Geometry: final body of the model. Coordinates: model frame, mm. Face numbers are marked on the shaded views. A direction names the side the tool comes from. Coordinates: 2 decimals unless noted, no trailing zeros. Order: outer loops, then holes, each group sorted by start corner. A loop starts at its lowest first (then second) coordinate and runs counter-clockwise, first axis right, second up. Notation, with made-up numbers: (64, -18) -> (95, -18) arc R30 ccw to (95, 8) -> close; hole circle Ø5 at (15, 56.5). An arc over 180 degrees is marked (long way). Answer in a Markdown table with one row per item. Add a question column.
1) Ray query, line 1 (Z direction, x = 45, y = 4); line 2 (X direction, y = 4.5, z = -26.5) (3 decimals); line 3 (Z direction, x = 63, y = 7.5). Return the intervals inside material, ascending. Write a range as from..to.
2) Section query A-A on x = 25. Return the cut outline in (y, z) (3 decimals).
3) Section query D-D on x = 48. Return the cut outline in (y, z) (3 decimals), then the cut area to 3 significant figures.
4) Section query B-B on y = 6.5. Return the cut outline in (x, z) (3 decimals), then the cut area to 3 significant figures.
5) Contact query for flat-ended pins moving along their axis: P1, Ø3.5, axis at y = 1, z = -11, coming from the -X side; P2, Ø2.5, axis at y = 1.5, z = -12, coming from the +X side; P3, Ø2.5, axis at x = 55.5, y = 1.5, coming from the +Z side; P4, Ø3.5, axis at y = 2.5, z = -13, coming from the -X side. Output: stop coordinate, or through.
6) Set-up query: the marked faces 1 and 2. Return all of +Z, -Z, +X, -X, +Y, -Y with unobstructed straight access to the full face (end or side cutting, diameter ignored); none if empty.
7) Section query C-C on z = -13. Return the cut outline in (x, y) (3 decimals), then the cut area to 3 significant figures.
8) Pull-direction query (Z, two-part tool) for the marked faces 3, 4 and 5; classes: +Z half, -Z half, draft (parallel to the pull), parting line (faces both ways), or undercut.
```python
from build123d import *

# Parameters (mm, degrees)
SKETCH1_W           = 72.39
SKETCH1_H           = 48.514
BOSS_EXTRUDE1_DEPTH = 8.636
SKETCH2_W           = 63.5
SKETCH2_H           = 40.64
CUT_EXTRUDE1_DEPTH  = 5.461
FILLET2_R           = 7.62
FILLET3_R           = 3.81
SKETCH4_R           = 2.25
SKETCH4_W           = 12.6
SKETCH4_H           = 5
SKETCH4_W_2         = 6.604
SKETCH4_H_2         = 6.604
CUT_EXTRUDE2_DEPTH  = 7.366
SKETCH5_R           = 1.35
SKETCH5_R_2         = 1.3499973
SKETCH5_R_3         = 1.385
SKETCH5_R_4         = 0.75
BOSS_EXTRUDE2_DEPTH = 7.366


with BuildPart() as part:
    # Sketch1 → Boss-Extrude1 (new body)
    with BuildSketch(Plane(origin=(0, 0, 0), x_dir=(1, 0, 0), z_dir=(0, 1, 0))):
        with Locations((36.195, 24.257)):
            Rectangle(SKETCH1_W, SKETCH1_H)
    extrude(amount=BOSS_EXTRUDE1_DEPTH)

    # Sketch2 → Cut-Extrude1 (cut)
    with BuildSketch(Plane(origin=(0, 8.636, 0), x_dir=(1, 0, 0), z_dir=(0, 1, 0))):
        with Locations((36.195, 24.257)):
            Rectangle(SKETCH2_W, SKETCH2_H)
    extrude(amount=-CUT_EXTRUDE1_DEPTH, mode=Mode.SUBTRACT)

    # Fillet2
    fillet2_edges = [part.edges().sort_by_distance(p)[0] for p in [
        (0, 4.318, -48.514),
        (72.39, 4.318, -48.514),
        (72.39, 4.318, 0),
        (0, 4.318, 0),
    ]]
    fillet(fillet2_edges, radius=FILLET2_R)

    # Fillet3
    fillet3_edges = [part.edges().sort_by_distance(p)[0] for p in [
        (36.195, 0, -48.514),
        (0, 0, -24.257),
        (72.39, 0, -24.257),
        (36.195, 0, 0),
        (2.231846327, 0, -46.282153673),
        (2.231846327, 0, -2.231846327),
        (70.158153673, 0, -2.231846327),
        (70.158153673, 0, -46.282153673),
    ]]
    fillet(fillet3_edges, radius=FILLET3_R)

    # Sketch4 → Cut-Extrude2 (cut)
    with BuildSketch(Plane(origin=(0, 3.175, 0), x_dir=(1, 0, 0), z_dir=(0, 1, 0))):
        with Locations((37.211, 11.811)):
            Circle(SKETCH4_R)
        with Locations((55.499, 11.557)):
            Rectangle(SKETCH4_W, SKETCH4_H)
        with Locations((24.765, 11.557)):
            Rectangle(SKETCH4_W_2, SKETCH4_H_2)
    extrude(amount=-CUT_EXTRUDE2_DEPTH, mode=Mode.SUBTRACT)

    # Sketch5 → Boss-Extrude2 (add)
    with BuildSketch(Plane(origin=(0, 3.175, 0), x_dir=(1, 0, 0), z_dir=(0, 1, 0))):
        with Locations((9.525, 39.497)):
            Circle(SKETCH5_R)
        with Locations((9.525, 9.017)):
            Circle(SKETCH5_R_2)
        with Locations((62.865, 39.497)):
            Circle(SKETCH5_R_3)
        with Locations((62.865, 9.017)):
            Circle(SKETCH5_R_4)
    extrude(amount=BOSS_EXTRUDE2_DEPTH)


solid = part.part
```
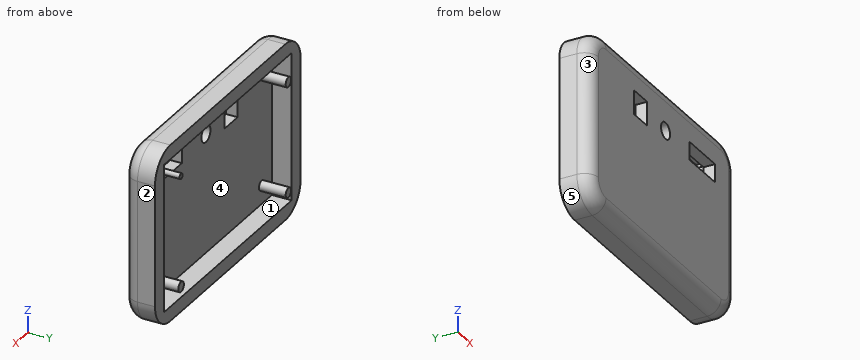
Result:
| question | item | result |
|---|---|---|
| 1 | line 1 | -48.51..-44.58, -3.94..0 |
| 1 | line 2 | 0..4.445, 67.945..72.39 |
| 1 | line 3 | -48.51..-44.58, -40.88..-38.12, -9.75..-8.28, -3.94..0 |
| 2 | outline | (0, -44.704) arc R3.81 ccw to (3.81, -48.514) -> (8.636, -48.514) -> (8.636, -44.577) -> (3.175, -44.577) -> (3.175, -14.859) -> (0, -14.859) -> close; (0, -8.255) -> (3.175, -8.255) -> (3.175, -3.937) -> (8.636, -3.937) -> (8.636, 0) -> (3.81, 0) arc R3.81 ccw to (0, -3.81) -> close |
| 3 | outline | (0, -44.704) arc R3.81 ccw to (3.81, -48.514) -> (8.636, -48.514) -> (8.636, -44.577) -> (3.175, -44.577) -> (3.175, -3.937) -> (8.636, -3.937) -> (8.636, 0) -> (3.81, 0) arc R3.81 ccw to (0, -3.81) -> close |
| 3 | area | 191 mm2 |
| 4 | outline | (0, -40.894) arc R7.62 ccw to (7.62, -48.514) -> (64.77, -48.514) arc R7.62 ccw to (72.39, -40.894) -> (72.39, -7.62) arc R7.62 ccw to (64.77, 0) -> (7.62, 0) arc R7.62 ccw to (0, -7.62) -> close; circle Ø2.7 at (9.525, -39.497); circle Ø2.7 at (9.525, -9.017); circle Ø2.77 at (62.865, -39.497); circle Ø1.5 at (62.865, -9.017); hole (4.445, -44.577) -> (67.945, -44.577) -> (67.945, -3.937) -> (4.445, -3.937) -> close |
| 4 | area | 901 mm2 |
| 5 | P1 | x = 0.15 |
| 5 | P2 | x = 72.24 |
| 5 | P3 | z = -0.15 |
| 5 | P4 | x = 0 |
| 6 | face 1 | +Y |
| 6 | face 2 | +Z, -Z, +X, +Y, -Y |
| 7 | outline | (0, 3.81) arc R3.81 ccw to (3.81, 0) -> (21.463, 0) -> (21.463, 3.175) -> (4.445, 3.175) -> (4.445, 8.636) -> (0, 8.636) -> close; (28.067, 0) -> (35.301, 0) -> (35.301, 3.175) -> (28.067, 3.175) -> close; (39.121, 0) -> (49.199, 0) -> (49.199, 3.175) -> (39.121, 3.175) -> close; (61.799, 0) -> (68.58, 0) arc R3.81 ccw to (72.39, 3.81) -> (72.39, 8.636) -> (67.945, 8.636) -> (67.945, 3.175) -> (61.799, 3.175) -> close |
| 7 | area | 199 mm2 |
| 8 | face 3 | draft |
| 8 | face 4 | undercut |
| 8 | face 5 | -Z half |
